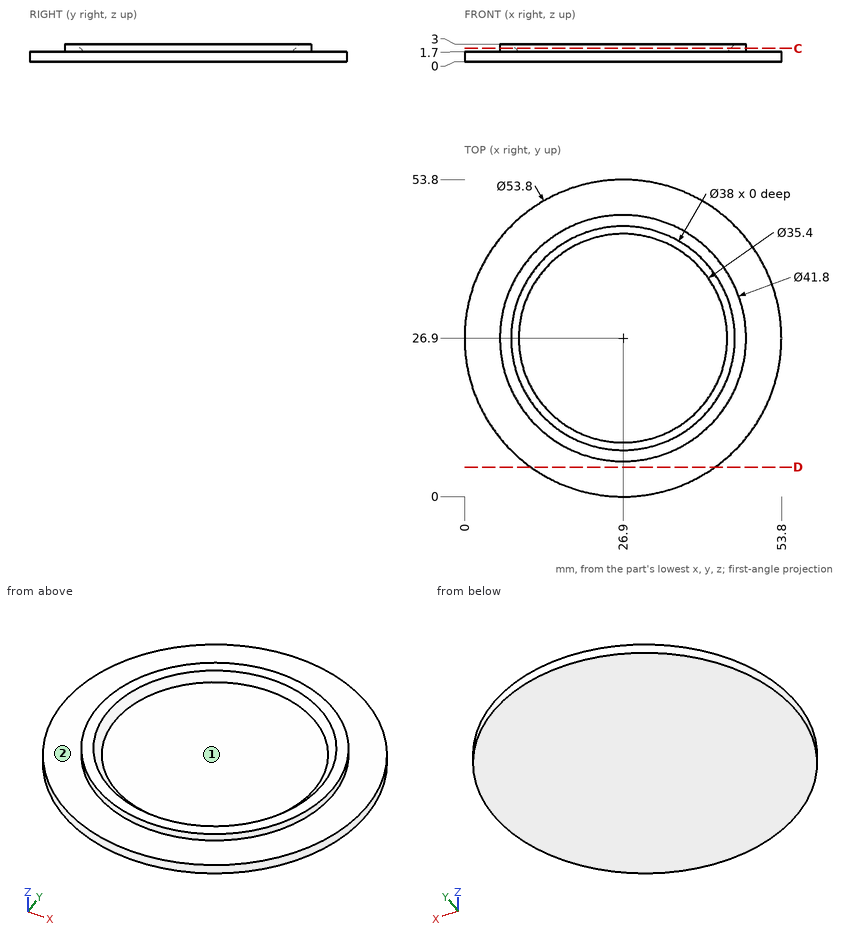
For this review, use the dimensioned drawing (mm, ordinates from the lowest corner) and the shaded views. Coordinates: 2 decimals unless noted, no trailing zeros. Write each loop counter-clockwise with the first axis right and the second up, starting at its lowest first coordinate (ties: lowest second). Pieces come first, ordered by that corner, then holes. Notation, with made-up numbers: (-37, -5.75) - (-8, -5.75) arc R9 cw to (-8, 4.25) - close; hole circle Ø6 at (43.5, 20). An arc over 180 degrees is marked (long way). One line per item, written item: value.
1) Mouldability with a two-part tool opening along Y and no side actions: class the marked faces 1 and 2 as +Y half, -Y half, draft (parallel to the pull), parting line (faces both ways), or undercut.
Answer sheet:
face 1: undercut
face 2: draft
2) Add section D-D (y = 5). State the section outline as (x, z) points.
Answer sheet:
outline: (11.28, 0) - (42.52, 0) - (42.52, 1.7) - (11.28, 1.7) - close
3) To check wall thickness, follow probe 1 along Z at (x, y) = (30, 6); probe 2 along X at (y, z) = (11, 1.9); probe 3 along Y at (x, z) = (15.5, 2.5). State the ranges of each line that lie inside material, in increasing order.
Answer sheet:
probe 1: z = 0 to 1.7
probe 2: x = 13.34 to 18.68, 35.12 to 40.46
probe 3: y = 9.38 to 12.33, 41.47 to 44.42
4) Insertion check: pin 1 (10 mm diameter, centred on x = 33.5, y = 25, fed in from +Z). The pin has a flat end and moves straight along its axis. Give the tip position at first contact, or say it passes through.
Answer sheet:
pin 1: stops at z = 1.7
5) Add section C-C (z = 2.25). State the section outline as (x, y) points.
Answer sheet:
outline: circle Ø41.8 at (26.9, 26.9); hole circle Ø36.5 at (26.9, 26.9)
